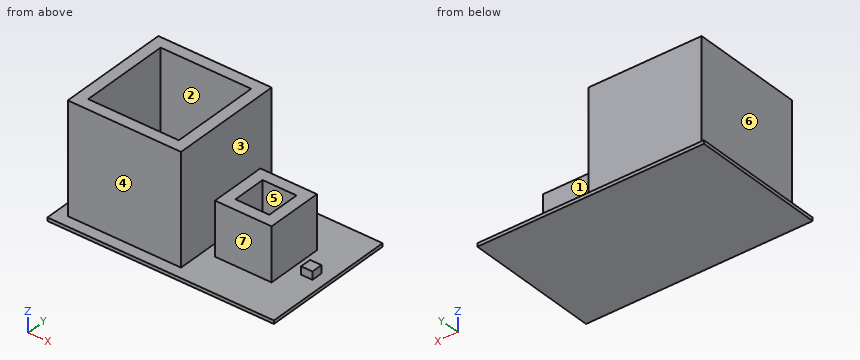
```python
from build123d import *

# Parameters (mm, degrees)
F0_W         = 10
F0_H         = 10
F1_DEPTH     = 10
F0_W_2       = 5
F0_H_2       = 5
F2_DEPTH     = 5
F0_W_3       = 1
F0_H_3       = 1
F3_DEPTH     = 1
F0_W_4       = 20
F0_H_4       = 12
F4_DEPTH     = 0.3
F5_T         = 1
F5_T3_DEPTH  = 3
F5_T5_DEPTH  = 12
F5_T7_DEPTH  = 12
F5_T9_DEPTH  = 7
F5_T11_DEPTH = 7
F5_T13_DEPTH = 3


# Not quite as in the source:
# - a shell that OpenCascade refuses in one call is made with other operations: the cavity is built on its own and cut out


with BuildPart() as f1:
    # F0 (on Top) → F1 (new body)
    with BuildSketch(Plane.XY):
        Rectangle(F0_W, F0_H)
    extrude(amount=F1_DEPTH)



with BuildPart() as f2:
    # F0 (on Top) → F2 (new body)
    with BuildSketch(Plane.XY):
        with Locations((8.5, 0)):
            Rectangle(F0_W_2, F0_H_2)
    extrude(amount=F2_DEPTH)


with BuildPart() as f3:
    # F0 (on Top) → F3 (new body)
    with BuildSketch(Plane.XY):
        with Locations((12.5, 0)):
            Rectangle(F0_W_3, F0_H_3)
    extrude(amount=F3_DEPTH)


with BuildPart() as f1_1:
    add(f1.part)

    add(f2.part)  # F4 merges F2

    add(f3.part)  # F4 merges F3
    # F0 (on Top) → F4 (join)
    with BuildSketch(Plane.XY):
        with Locations((4, 0)):
            Rectangle(F0_W_4, F0_H_4)
        Rectangle(F0_W, F0_H, mode=Mode.SUBTRACT)
        with Locations((8.5, 0)):
            Rectangle(F0_W_2, F0_H_2, mode=Mode.SUBTRACT)
        with Locations((12.5, 0)):
            Rectangle(F0_W_3, F0_H_3, mode=Mode.SUBTRACT)
    extrude(amount=F4_DEPTH)

    # F5: shell of thickness 1, made by hand


with BuildPart() as f5_core1:
    # F5_t2: copy of F1
    add(f1_1.part)

    # the walls: a layer under each face that stays
    f5_faces = [f5_core1.faces().sort_by_distance(p)[0] for p in [
        (13, 0, 0.65),
        (10.6666666667, -4, 0.3),
        (12.5, 0.5, 0.65),
        (12.5, -0.5, 0.65),
        (4, 6, 0.15),
        (-6, 0, 0.15),
        (4, -6, 0.15),
        (14, 0, 0.15),
        (0, 5, 5.15),
        (5, 0, 5.15),
        (0, -5, 5.15),
        (-5, 0, 5.15),
        (8.5, 2.5, 2.65),
        (11, 0, 2.65),
        (8.5, -2.5, 2.65),
        (6, 0, 2.65),
        (12, 0, 0.65),
        (4, 0, 0),
    ]]
    thicken(f5_faces, amount=-F5_T, mode=Mode.SUBTRACT)

    # F5_s4 → F5_t3 (cut)
    with BuildSketch(Plane.XZ.offset(-1.5)):
        Polygon((13.01, 0.31), (12, 0.3), (12, -0.7), (13, -0.7), align=None)
        Polygon((11.99, 0.31), (12, -0.7), (13, -0.7), (13, 0.3), align=None)
    extrude(amount=F5_T3_DEPTH, mode=Mode.SUBTRACT)

    # F5_s6 → F5_t5 (cut)
    with BuildSketch(Plane.YZ.offset(-6)):
        Polygon((5.01, 0.31), (5, -0.7), (4, -0.7), (4, 0.3), align=None)
        Polygon((-5.01, 0.31), (-5, -0.7), (-4, -0.7), (-4, 0.3), align=None)
    extrude(amount=F5_T5_DEPTH, mode=Mode.SUBTRACT)

    # F5_s8 → F5_t7 (cut)
    with BuildSketch(Plane.XZ.offset(-6)):
        Polygon((5.01, 0.31), (5, -0.7), (4, -0.7), (4, 0.3), align=None)
        Polygon((-5.01, 0.31), (-5, -0.7), (-4, -0.7), (-4, 0.3), align=None)
    extrude(amount=F5_T7_DEPTH, mode=Mode.SUBTRACT)

    # F5_s10 → F5_t9 (cut)
    with BuildSketch(Plane.YZ.offset(5)):
        Polygon((2.51, 0.31), (2.5, -0.7), (1.5, -0.7), (1.5, 0.3), align=None)
        Polygon((-2.51, 0.31), (-2.5, -0.7), (-1.5, -0.7), (-1.5, 0.3), align=None)
    extrude(amount=F5_T9_DEPTH, mode=Mode.SUBTRACT)

    # F5_s12 → F5_t11 (cut)
    with BuildSketch(Plane.XZ.offset(-3.5)):
        Polygon((11.01, 0.31), (11, -0.7), (10, -0.7), (10, 0.3), align=None)
        Polygon((5.99, 0.31), (6, -0.7), (7, -0.7), (7, 0.3), align=None)
    extrude(amount=F5_T11_DEPTH, mode=Mode.SUBTRACT)

    # F5_s14 → F5_t13 (cut)
    with BuildSketch(Plane.YZ.offset(11)):
        Polygon((0.51, 0.31), (0.5, -0.7), (-0.5, -0.7), (-0.5, 0.3), align=None)
        Polygon((-0.51, 0.31), (-0.5, -0.7), (0.5, -0.7), (0.5, 0.3), align=None)
    extrude(amount=F5_T13_DEPTH, mode=Mode.SUBTRACT)


with BuildPart() as f1_2:
    add(f1_1.part)

    # what is left inside the walls is the cavity
    f5_cavity = [f5_core1.part.solids().sort_by_distance(p)[0] for p in [
        (3.99, 0, 7),
        (8.5, 1.49, 3.666667),
    ]]
    add(f5_cavity, mode=Mode.SUBTRACT)


solid = f1_2.part
```
Geometry check sheet. Reference: the model listing, model coordinates, mm. Face numbers are marked on the shaded views. A direction names the side the tool comes from. Coordinates: 2 decimals unless noted, no trailing zeros. Order: outer loops, then holes, each group sorted by start corner. A loop starts at its lowest first (then second) coordinate and runs counter-clockwise, first axis right, second up. Notation, with made-up numbers: M 7,41 L 46,41 A26 cw 46,70 Z; hole C -18,-12.5 d1. An arc over 180 degrees is marked long. Answer as a JSON object with one key per item and string values.
Q1. Depth check by flat-ended pin: pin 1 Ø1.5 at (y, z) = (-4.5, 6.5) entering from +X; pin 2 Ø1 at (x, z) = (10.5, 4.5) entering from -Y; pin 3 Ø5 at (x, z) = (7.5, 2.5) entering from +Y; pin 4 Ø3.5 at (x, y) = (9, -0.5) entering from +Z. Enter the tip coordinate at first touch or a pass-through.
Results are:
{"pin 1": "stops at x = 5", "pin 2": "stops at y = -2.5", "pin 3": "stops at y = 6", "pin 4": "stops at z = 5"}
Q2. Cross-section at C-C on y = 2.25. Record the cut outline in (x, z), and give its area (3 significant figures).
Results are:
{"outline": "M -6,0 L 14,0 L 14,0.3 L 11,0.3 L 11,5 L 6,5 L 6,0.3 L 5,0.3 L 5,10 L 4,10 L 4,1 L -4,1 L -4,10 L -5,10 L -5,0.3 L -6,0.3 Z", "area": "54.5 mm²"}
Q3. Release check for a two-part mould opening along X. For the marked faces 5, 6 and 7 record: released by +X, released by -X, zero draft, split by the parting line, or undercut.
Results are:
{"face 5": "undercut", "face 6": "released by -X", "face 7": "zero draft"}
Q4. Cross-section at A-A on z = 1.25. Record the cut outline in (x, y), and give its area (3 significant figures).
Results are:
{"outline": "M -5,-5 L 5,-5 L 5,5 L -5,5 Z; M 6,-2.5 L 11,-2.5 L 11,2.5 L 6,2.5 Z; hole M -4,-4 L 4,-4 L 4,4 L -4,4 Z; hole M 7,-1.5 L 10,-1.5 L 10,1.5 L 7,1.5 Z", "area": "52.0 mm²"}
Q5. Cross-section at D-D on z = 6.5. Record the cut outline in (x, y).
Results are:
{"outline": "M -5,-5 L 5,-5 L 5,5 L -5,5 Z; hole M -4,-4 L 4,-4 L 4,4 L -4,4 Z"}
Q6. Tool access check on the marked faces 1, 2, 3 and 4. Record the directions out of +Z, -Z, +X, -X, +Y, -Y that give a thin tool (end or side, any length) a straight path to the whole face; none if there is none.
Results are:
{"face 1": "+Z, +X, +Y", "face 2": "+Z", "face 3": "+Z, +Y, -Y", "face 4": "+Z, +X, -X, -Y"}
Q7. Scan lines: line 1 (X direction, y = 1.25, z = 6.75); line 2 (Y direction, x = 8.5, z = 3.5). Record each from-to range of solid material in increasing order.
Results are:
{"line 1": "x = -5 to -4, 4 to 5", "line 2": "y = -2.5 to -1.5, 1.5 to 2.5"}
Q8. Cross-section at B-B on x = 9.75. Record the cut outline in (y, z).
Results are:
{"outline": "M -6,0 L 6,0 L 6,0.3 L 2.5,0.3 L 2.5,5 L 1.5,5 L 1.5,1 L -1.5,1 L -1.5,5 L -2.5,5 L -2.5,0.3 L -6,0.3 Z"}
